```python
from build123d import *

# Parameters (mm, degrees)
F0_W     = 17.4
F0_H     = 8.8
F0_W_2   = 13.4
F0_H_2   = 6.2
F1_DEPTH = 10
F2_W     = 17.4
F2_H     = 10
F3_DEPTH = 4
F4_D     = 4.6
F4_DEPTH = 10
F4_TIP   = 1.3819794238
F5_R     = 5
F6_SIZE  = 0.6


# Not quite as in the source:
# - a feature names something its author has since deleted; it is built from what else it names


with BuildPart() as f1:
    # F0 (on Top) → F1 (new body)
    with BuildSketch(Plane.XY):
        with Locations((-5.3887722373, 2.3212898893)):
            Rectangle(F0_W, F0_H)
        with Locations((-5.3887722373, 3.0212898893)):
            Rectangle(F0_W_2, F0_H_2, mode=Mode.SUBTRACT)
    extrude(amount=F1_DEPTH)

    # F2 (on face) → F3 (join)
    with BuildSketch(Plane(origin=(0, 6.7212898893, 0), x_dir=(-1, 0, 0), z_dir=(0, 1, 0))):
        with Locations((5.3887722373, 5)):
            Rectangle(F2_W, F2_H)
        Polygon((-3.3112277627, 0), (-3.3112277627, 10), (-16.2704663397, -20.530052861), (2.069760485, -28.3150172716), (14.0887722373, 0), align=None)
    extrude(amount=F3_DEPTH)

    # F4
    with Locations(Plane(origin=(0, 6.7212898893, 0), x_dir=(-1, 0, 0), z_dir=(0, -1, 0))):
        with Locations((0.1372122432, 7.4690311061), (-4.5515612986, 18.5150893475)):
            Hole(F4_D / 2, depth=F4_DEPTH)
            with Locations((0, 0, -(F4_DEPTH + F4_TIP / 2))):  # 118° drill point
                Cone(0, F4_D / 2, F4_TIP, mode=Mode.SUBTRACT)

    # F5
    f5_edges = [f1.edges().sort_by_distance(p)[0] for p in [
        (16.270466, 8.72129, -20.530053),
        (-2.06976, 8.72129, -28.315017),
    ]]
    fillet(f5_edges, radius=F5_R)

    # F6
    f6_edges = [f1.edges().sort_by_distance(p)[0] for p in [
        (-5.388772, 6.12129, 10),
        (1.311228, 3.02129, 10),
        (-12.088772, 3.02129, 10),
        (-5.388772, -0.07871, 10),
    ]]
    chamfer(f6_edges, length=F6_SIZE)


solid = f1.part
```
Verification items for the finished model (mm, model axes). A direction names the side the tool comes from. Coordinates: 2 decimals unless noted, no trailing zeros. Loops run counter-clockwise (first coordinate to the right, second up) from the corner with the lowest first, then second, coordinate; pieces in that order, holes last. Notation, with made-up numbers: (72.5, 26) -> (76.5, 26) arc R30 ccw to (76.5, 58) -> close; hole circle Ø2 at (11.25, 36). An arc over 180 degrees is marked (long way). Answer in a Markdown table with one row per item.
1) Section check C-C (y = 9.5). Record the cut outline in (x, z).
The answers:
| item | result |
|---|---|
| outline | (-14.09, 0) -> (-4.02, -23.71) arc R5 ccw to (2.53, -26.36) -> (11.67, -22.48) arc R5 ccw to (14.32, -15.93) -> (3.31, 10) -> (-14.09, 10) -> close; hole circle Ø4.6 at (-0.14, -7.47); hole circle Ø4.6 at (4.55, -18.52) |
2) Section check A-A (y = 0.75). Record the cut outline in (x, z), and give its area (3 significant figures).
The answers:
| item | result |
|---|---|
| outline | (-14.09, 0) -> (-12.09, 0) -> (-12.09, 9.4) -> (-12.69, 10) -> (-14.09, 10) -> close; (1.31, 0) -> (3.31, 0) -> (3.31, 10) -> (1.91, 10) -> (1.31, 9.4) -> close |
| area | 39.6 mm2 |
3) Scan lines: line 1 along X through (y, z) = (3, 4.5); line 2 along Y through (x, z) = (12.5, -22); line 3 along X through (y, z) = (-1.5, 7). Record each from-to range of solid material in increasing order. Write a range as from..to.
The answers:
| item | result |
|---|---|
| line 1 | x = -14.09..-12.09, 1.31..3.31 |
| line 2 | y = 6.72..10.72 |
| line 3 | x = -14.09..3.31 |
4) Section check D-D (z = 1). Record the cut outline in (x, y).
The answers:
| item | result |
|---|---|
| outline | (-14.09, -2.08) -> (3.31, -2.08) -> (3.31, 6.72) -> (7.13, 6.72) -> (7.13, 10.72) -> (-14.09, 10.72) -> close; hole (-12.09, -0.08) -> (1.31, -0.08) -> (1.31, 6.12) -> (-12.09, 6.12) -> close |
5) Section check B-B (x = -8.5). Record the cut outline in (y, z), and give its area (3 significant figures).
The answers:
| item | result |
|---|---|
| outline | (-2.08, 0) -> (-0.08, 0) -> (-0.08, 9.4) -> (-0.68, 10) -> (-2.08, 10) -> close; (6.12, 0) -> (6.72, 0) -> (6.72, -13.17) -> (10.72, -13.17) -> (10.72, 10) -> (6.72, 10) -> (6.12, 9.4) -> close |
| area | 118 mm2 |
6) Depth check by flat-ended pin: P1, Ø8, axis at x = 10.5, z = -8, coming from the -Y side; P2, Ø3, axis at y = 8.5, z = -12, coming from the -X side; P3, Ø3.5, axis at x = 4.55, z = -18.52, coming from the +Y side; P4, Ø4.5, axis at y = 3, z = 3, coming from the +X side. Enter the tip coordinate at first touch or a pass-through.
The answers:
| item | result |
|---|---|
| P1 | stops at y = 6.72 |
| P2 | stops at x = -9.63 |
| P3 | passes through |
| P4 | stops at x = 3.31 |
7) Access from +Z, -Z, +X, -X, +Y, -Y to the whole of each face (thin tool, end or side, straight path). Record for faces 4 (the face through (3.311, 2, 5)), 5 (the face through (-5, -0.079, 5)), 6 (the face through (-0.636, 8.749, -5.224)), 7 (the face through (-8.986, 8.693, -12.022)), 8 (the face through (-6, -1, 0)).
The answers:
| item | result |
|---|---|
| face 4 | +Z, -Z, +X, -Y |
| face 5 | +Z, -Z |
| face 6 | +Y, -Y |
| face 7 | -Z, -X, +Y, -Y |
| face 8 | -Z, +X, -X, -Y |
8) Draft check along Y on faces 1 (the face through (-6, -2.079, 5)), 2 (the face through (-3, 10.721, -8)), 3 (the face through (-12.089, 3, 5)). Enter one of: released by +Y, released by -Y, zero draft, split by the parting line, or undercut.
The answers:
| item | result |
|---|---|
| face 1 | released by -Y |
| face 2 | released by +Y |
| face 3 | undercut |
